from build123d import *

# Parameters (mm, degrees)
SKETCH1_W                        = 38.1
SKETCH1_H                        = 38.1
SKETCH1_W_2                      = 31.75
SKETCH1_H_2                      = 31.75
BOSS_EXTRUDE1_DEPTH              = 374.65
F_25_64_0_39063_DIAMETER_HOLE1_D = 9.922002


with BuildPart() as part:
    # Sketch1 → Boss-Extrude1 (new body)
    with BuildSketch(Plane.XY):
        Rectangle(SKETCH1_W, SKETCH1_H)
        Rectangle(SKETCH1_W_2, SKETCH1_H_2, mode=Mode.SUBTRACT)
    extrude(amount=BOSS_EXTRUDE1_DEPTH)

    # 25/64 (0.39063) Diameter Hole1 (through all)
    with Locations(Plane(origin=(0, 19.05, 0), x_dir=(1, 0, 0), z_dir=(0, 1, 0))):
        with Locations((0, -187.325)):
            Hole(F_25_64_0_39063_DIAMETER_HOLE1_D / 2)


solid = part.part
Design review of the part built by this model. Coordinates are the model's own, in mm. A direction names the side the tool comes from. Round coordinates to 2 decimals unless told otherwise and drop trailing zeros. Loops run counter-clockwise (first coordinate to the right, second up) from the corner with the lowest first, then second, coordinate; pieces in that order, holes last. Notation, with made-up numbers: (9, -34) - (63, -34) arc R11 cw to (63, -27) - close; hole circle Ø7 at (2.5, 46.25). An arc over 180 degrees is marked (long way). One line per item, written item: value. Start each with the question number.
1) Draft analysis for pull direction Z (two halves, no side actions). For faces 3 (the cylindrical face through (0.6, 17.4, 182.4)), 4 (the flat face through (7, 15.875, 185)), 5 (the flat face through (-17, 0, 374.65)), state which applies: +Z half, -Z half, draft (parallel to the pull), parting line (faces both ways), or undercut.
2) Consider section B-B on z = 227.5. Give the boundary of the cut face in (x, y) (3 decimals), then the cut area to 3 significant figures.
3) Consider section A-A on x = 0. Give the boundary of the cut face in (y, z) (3 decimals), then the cut area to 3 significant figures.
4) To check wall thickness, follow L1, parallel to X at y = 2, z = 177 (3 decimals); L2, parallel to Z at x = 0, y = -17.15. State the ranges of each line that lie inside material, in increasing order. Write a range as from..to.
5) For faces 1 (the flat face through (-19.05, 0, 185)), 2 (the flat face through (15.875, 0, 185)), list the 3-axis set-ups (+Z, -Z, +X, -X, +Y, -Y) from which the entire face can be reached by the end or side of a thin tool; tool diameter is ignored.
Reported:
1. face 3: undercut
1. face 4: draft
1. face 5: +Z half
2. outline: (-19.05, -19.05) - (19.05, -19.05) - (19.05, 19.05) - (-19.05, 19.05) - close; hole (-15.875, -15.875) - (15.875, -15.875) - (15.875, 15.875) - (-15.875, 15.875) - close
2. area: 444 mm^2
3. outline: (-19.05, 0) - (-15.875, 0) - (-15.875, 182.364) - (-19.05, 182.364) - close; (-19.05, 192.286) - (-15.875, 192.286) - (-15.875, 374.65) - (-19.05, 374.65) - close; (15.875, 0) - (19.05, 0) - (19.05, 182.364) - (15.875, 182.364) - close; (15.875, 192.286) - (19.05, 192.286) - (19.05, 374.65) - (15.875, 374.65) - close
3. area: 2,320 mm^2
4. L1: x = -19.05..-15.875, 15.875..19.05
4. L2: z = 0..182.36, 192.29..374.65
5. face 1: +Z, -Z, -X, +Y, -Y
5. face 2: +Z, -Z
